```python
from build123d import *

# Parameters (mm, degrees)
F0_R     = 38.1
F1_DEPTH = 76.2
F2_W     = 25.4
F2_H     = 12.7
F3_DEPTH = 63.5
F4_R     = 6.35
F5_R     = 31.75
F6_DEPTH = 76.201


with BuildPart() as f1:
    # F0 (on Top) → F1 (new body)
    with BuildSketch(Plane.XY):
        Circle(F0_R)
    extrude(amount=F1_DEPTH)

    # F2 (on Front) → F3 (cut, symmetric)
    with BuildSketch(Plane.XZ):
        Rectangle(F2_W, F2_H)
    extrude(amount=F3_DEPTH, both=True, mode=Mode.SUBTRACT)

    # F4
    f4_edges = [f1.edges().sort_by_distance(p)[0] for p in [
        (0, 38.1, 6.35),
        (0, -38.1, 6.35),
    ]]
    fillet(f4_edges, radius=F4_R)

    # F5 (on face) → F6 (cut, through all)
    with BuildSketch(Plane(origin=(0, 0, 0), x_dir=(1, 0, 0), z_dir=(0, 0, -1))):
        Circle(F5_R)
    extrude(amount=-F6_DEPTH, mode=Mode.SUBTRACT)


solid = f1.part
```
The listing builds one solid part. Answer for the finished solid, in the listing's coordinates (mm). Give positions to 0.01 mm unless a question says otherwise; leave off trailing zeros. Order: outer loops, then holes, each group sorted by start corner. A loop starts at its lowest first (then second) coordinate and runs counter-clockwise, first axis right, second up. Notation, with made-up numbers: (79, 53) -> (119, 53) arc R6 ccw to (119, 61) -> close; hole circle Ø8 at (42, 31.5). An arc over 180 degrees is marked (long way). Answer as a JSON object with one key per item and string values. Group by question number.
Item 1: Determine the mould class of faces 1 (the cylindrical face through (29.33, 12.16, 37.57)), 2 (the cylindrical face through (36.34, 11.44, 37.57)), 3 (the flat face through (-32, -2, 0)) for opening direction Y: pulls with the +Y half, pulls with the -Y half, needs draft (parallel to the pull), parting line crosses it, or undercut.
Item 2: Consider L1, parallel to Y at x = 0, z = 32.5; L2, parallel to X at y = -8, z = 8.5. Determine where each line is inside the solid, lowest interval first. Write a range as from..to.
Item 3: The part is cut by section B-B on x = 0. Write down the section's boundary in (y, z).
Item 4: The part is cut by section A-A on y = 0. Write down the section's boundary in (x, z).
Item 5: The part is cut by section C-C on z = 50. Write down the section's boundary in (x, y).
Item 6: Flat-ended cylindrical pins translate along their axes: pin 1 (3.5 mm diameter, centred on y = -31, z = 7, fed in from +X); pin 2 (10 mm diameter, centred on y = -12, z = 42.5, fed in from -X); pin 3 (12 mm diameter, centred on x = 14, z = 17, fed in from +Y). Find the tip coordinate at first contact, or state that the pin passes through.
Result set:
{
 "1": {"face 1": "undercut", "face 2": "parting line crosses it", "face 3": "needs draft"},
 "2": {"L1": "-38.1..-31.75, 31.75..38.1", "L2": "-37.25..-30.73, 30.73..37.25"},
 "3": {"outline": "(-38.1, 12.7) arc R6.35 ccw to (-31.75, 6.35) -> (-31.75, 76.2) -> (-38.1, 76.2) -> close; (31.75, 6.35) arc R6.35 ccw to (38.1, 12.7) -> (38.1, 76.2) -> (31.75, 76.2) -> close"},
 "4": {"outline": "(-38.1, 0) -> (-31.75, 0) -> (-31.75, 76.2) -> (-38.1, 76.2) -> close; (31.75, 0) -> (38.1, 0) -> (38.1, 76.2) -> (31.75, 76.2) -> close"},
 "5": {"outline": "circle Ø76.2 at (0, 0); hole circle Ø63.5 at (0, 0)"},
 "6": {"pin 1": "x = 24.41", "pin 2": "x = -37.45", "pin 3": "y = 37.25"}
}
